CAD build for the part. Positions are in the model's coordinates, mm. A direction names the side the tool comes from. Give positions to 0.01 mm unless a question says otherwise; leave off trailing zeros. Write each loop counter-clockwise with the first axis right and the second up, starting at its lowest first coordinate (ties: lowest second). Pieces come first, ordered by that corner, then holes. Notation, with made-up numbers: (18, -36.5) - (58, -36.5) arc R19 ccw to (58, -7.5) - close; hole circle Ø1 at (17, 29). An arc over 180 degrees is marked (long way). Put each result on its own line as item: value. Start each with the question number.
1. Cut at A-A on x = 0. List the corners of the cut face in (y, z).
2. Cut at D-D on x = -32. List the corners of the cut face in (y, z).
3. Wall check: line 1 (Y direction, x = 0, z = 1.7); line 2 (X direction, y = -10, z = 3.35); line 3 (Y direction, x = 33, z = 2.85). Give the ranges that are in metal, low to high.
4. Mould opens along X. For faces 1 (the cylindrical face through (-0.56, -44.54, 2.46)), 2 (the cylindrical face through (60.14, -39.1, 2.54)), 3 (the flat face through (41, 40, 2)) say: +X half, -X half, draft (parallel to the pull), parting line (faces both ways), or undercut.
5. Drop flat-ended pins along their axis: pin 1 (18 mm diameter, centred on x = -12, y = 14, fed in from +Z); pin 2 (1.5 mm diameter, centred on x = 42.5, z = 2, fed in from +Y); pin 3 (3 mm diameter, centred on x = -9.5, z = 3.5, fed in from +Y); pin 4 (4.5 mm diameter, centred on x = 0, y = 42, fed in from +Z). Give the stop position or say it passes through.
6. Cut at C-C on y = -42. List the corners of the cut face in (x, z), and give its area (3 significant figures).
7. Cut at B-B on z = 2.25. Give the number of separate pieces and of enclosed holes in the cut face, and give its area (3 significant figures).
8. Tool access for faces 4 (the flat face through (1, 1, 0)), 5 (the flat face through (-42, 40, 2)), 6 (the flat face through (-1, 30, 3)): list every direction of +Z, -Z, +X, -X, +Y, -Y with a clear straight run to the whole face (end or side of a thin tool).
from build123d import *

# Parameters (mm, degrees)
BOSS_EXTRUDE1_DEPTH  = 5
CUT_EXTRUDE1_START   = -10
SKETCH3_R            = 2.6
CUT_EXTRUDE1_DEPTH   = 10
FILLET1_R            = 10
FILLET2_R            = 3
SKETCH4_R            = 2.6
CUT_EXTRUDE2_DEPTH   = 10
CUT_EXTRUDE3_DEPTH   = 4
CUT_EXTRUDE4_DEPTH   = 83.286086309
MIRROR2_COPY_1_DEPTH = 83.286086309


with BuildPart() as part:
    # Sketch1 → Boss-Extrude1 (new body)
    with BuildSketch(Plane.XY):
        with BuildLine():
            Line((-58, 55), (58, 55))
            ThreePointArc((58, 55), (60.121320344, 54.121320344), (61, 52))
            Line((61, 52), (61, -52))
            ThreePointArc((61, -52), (60.121320344, -54.121320344), (58, -55))
            Line((58, -55), (-58, -55))
            ThreePointArc((-58, -55), (-60.121320344, -54.121320344), (-61, -52))
            Line((-61, -52), (-61, 52))
            ThreePointArc((-61, 52), (-60.121320344, 54.121320344), (-58, 55))
        make_face()
    extrude(amount=BOSS_EXTRUDE1_DEPTH)

    # Sketch3 → Cut-Extrude1 (cut)
    with BuildSketch(Plane.XY.offset(5).offset(CUT_EXTRUDE1_START)):
        with BuildLine():
            Line((-58, 55), (-8.6, 55))
            Line((-8.6, 55), (-8.6, 59.373865289))
            Line((-8.6, 59.373865289), (-61, 59.373865289))
            Line((-61, 59.373865289), (-61, 52))
            ThreePointArc((-61, 52), (-60.121320344, 54.121320344), (-58, 55))
        make_face()
        with BuildLine():
            Line((-17.597879381, 43.752948644), (-8.6, 55))
            Line((-8.6, 55), (-58, 55))
            ThreePointArc((-58, 55), (-60.121320344, 54.121320344), (-61, 52))
            Line((-61, 52), (-61, 40))
            Line((-61, 40), (-25.40648677, 40))
            ThreePointArc((-25.40648677, 40), (-21.074657685, 40.986939655), (-17.597879381, 43.752948644))
        make_face()
        with BuildLine():
            ThreePointArc((58, 55), (60.121320344, 54.121320344), (61, 52))
            Line((61, 52), (61, 59.373865289))
            Line((61, 59.373865289), (8.6, 59.373865289))
            Line((8.6, 59.373865289), (8.6, 55))
            Line((8.6, 55), (13.480832282, 55))
            Line((13.480832282, 55), (58, 55))
        make_face()
        with BuildLine():
            ThreePointArc((17.597879381, 43.752948644), (21.074657685, 40.986939655), (25.40648677, 40))
            Line((25.40648677, 40), (61, 40))
            Line((61, 40), (61, 52))
            ThreePointArc((61, 52), (60.121320344, 54.121320344), (58, 55))
            Line((58, 55), (13.480832282, 55))
            Line((13.480832282, 55), (8.6, 55))
            Line((8.6, 55), (17.597879381, 43.752948644))
        make_face()
        with BuildLine():
            Line((61, -52), (61, -40))
            Line((61, -40), (25.40648677, -40))
            ThreePointArc((25.40648677, -40), (21.074657685, -40.986939655), (17.597879381, -43.752948644))
            Line((17.597879381, -43.752948644), (8.6, -55))
            Line((8.6, -55), (58, -55))
            ThreePointArc((58, -55), (60.121320344, -54.121320344), (61, -52))
        make_face()
        with BuildLine():
            Line((61, -59.373865289), (61, -52))
            ThreePointArc((61, -52), (60.121320344, -54.121320344), (58, -55))
            Line((58, -55), (8.6, -55))
            Line((8.6, -55), (8.6, -59.373865289))
            Line((8.6, -59.373865289), (61, -59.373865289))
        make_face()
        with BuildLine():
            Line((-58, -55), (-8.6, -55))
            Line((-8.6, -55), (-17.597879381, -43.752948644))
            ThreePointArc((-17.597879381, -43.752948644), (-21.074657685, -40.986939655), (-25.40648677, -40))
            Line((-25.40648677, -40), (-61, -40))
            Line((-61, -40), (-61, -52))
            ThreePointArc((-61, -52), (-60.121320344, -54.121320344), (-58, -55))
        make_face()
        with BuildLine():
            Line((-8.6, -59.373865289), (-8.6, -55))
            Line((-8.6, -55), (-58, -55))
            ThreePointArc((-58, -55), (-60.121320344, -54.121320344), (-61, -52))
            Line((-61, -52), (-61, -59.373865289))
            Line((-61, -59.373865289), (-8.6, -59.373865289))
        make_face()
        with Locations((0, -42)):
            Circle(SKETCH3_R)
    extrude(amount=CUT_EXTRUDE1_DEPTH, mode=Mode.SUBTRACT)

    # Fillet1
    fillet1_edges = [part.edges().sort_by_distance(p)[0] for p in [
        (-8.6, 55, 2.5),
        (8.6, 55, 2.5),
        (8.6, -55, 2.5),
        (-8.6, -55, 2.5),
    ]]
    fillet(fillet1_edges, radius=FILLET1_R)

    # Fillet2
    fillet2_edges = [part.edges().sort_by_distance(p)[0] for p in [
        (-61, -40, 2.5),
        (-61, 40, 2.5),
        (61, 40, 2.5),
        (61, -40, 2.5),
    ]]
    fillet(fillet2_edges, radius=FILLET2_R)

    # Sketch4 → Cut-Extrude2 (cut)
    with BuildSketch(Plane.XY.offset(5)):
        with Locations((0, 42)):
            Circle(SKETCH4_R)
    extrude(amount=-CUT_EXTRUDE2_DEPTH, mode=Mode.SUBTRACT)

    # Sketch5 → Cut-Extrude3 (cut)
    with BuildSketch(Plane.XY.offset(5)):
        with BuildLine():
            Line((-46, 30), (46, 30))
            ThreePointArc((46, 30), (49.535533906, 28.535533906), (51, 25))
            Line((51, 25), (51, -25))
            ThreePointArc((51, -25), (49.535533906, -28.535533906), (46, -30))
            Line((46, -30), (-46, -30))
            ThreePointArc((-46, -30), (-49.535533906, -28.535533906), (-51, -25))
            Line((-51, -25), (-51, 25))
            ThreePointArc((-51, 25), (-49.535533906, 28.535533906), (-46, 30))
        make_face()
    extrude(amount=-CUT_EXTRUDE3_DEPTH, mode=Mode.SUBTRACT)

    # Sketch6 → Cut-Extrude4 (cut, through all)
    with BuildSketch(Plane(origin=(0, 0, 0), x_dir=(-1, 0, 0), z_dir=(0, 0, -1))):
        with BuildLine():
            Line((0, 50), (-7.785066229, 50))
            ThreePointArc((-7.785066229, 50), (-12.116895314, 49.013060345), (-15.593673618, 46.247051356))
            Line((-15.593673618, 46.247051356), (-17.583467028, 43.759875465))
            ThreePointArc((-17.583467028, 43.759875465), (-21.066662425, 40.988761251), (-25.40648677, 40))
            Line((-25.40648677, 40), (-25.40648677, 70))
            Line((-25.40648677, 70), (0, 70))
            Line((0, 70), (0, 50))
        make_face()
    cut_extrude4 = extrude(amount=-CUT_EXTRUDE4_DEPTH, mode=Mode.SUBTRACT)

    # Mirror1: Cut-Extrude4 across plane
    add(cut_extrude4.mirror(Plane(origin=(0, 0, 0), x_dir=(0, 0, 1), z_dir=(1, 0, 0))), mode=Mode.SUBTRACT)

    # Mirror2: Cut-Extrude4 across plane
    add(cut_extrude4.mirror(Plane.ZX), mode=Mode.SUBTRACT)

    # Mirror2 copy 1 sketch → Mirror2 copy 1 (cut, through all)
    with BuildSketch(Plane(origin=(0, 0, 0), x_dir=(1, 0, 0), z_dir=(0, 0, -1))):
        with BuildLine():
            Line((0, 50), (-7.785066229, 50))
            ThreePointArc((-7.785066229, 50), (-12.116895314, 49.013060345), (-15.593673618, 46.247051356))
            Line((-15.593673618, 46.247051356), (-17.583467028, 43.759875465))
            ThreePointArc((-17.583467028, 43.759875465), (-21.066662425, 40.988761251), (-25.40648677, 40))
            Line((-25.40648677, 40), (-25.40648677, 70))
            Line((-25.40648677, 70), (0, 70))
            Line((0, 70), (0, 50))
        make_face()
    extrude(amount=-MIRROR2_COPY_1_DEPTH, mode=Mode.SUBTRACT)


solid = part.part
Report:
1. outline: (-50, 0) - (-44.6, 0) - (-44.6, 5) - (-50, 5) - close; (-39.4, 0) - (39.4, 0) - (39.4, 5) - (30, 5) - (30, 1) - (-30, 1) - (-30, 5) - (-39.4, 5) - close; (44.6, 0) - (50, 0) - (50, 5) - (44.6, 5) - close
2. outline: (-40, 0) - (40, 0) - (40, 5) - (30, 5) - (30, 1) - (-30, 1) - (-30, 5) - (-40, 5) - close
3. line 1: y = -50 to -44.6, -39.4 to -30, 30 to 39.4, 44.6 to 50
3. line 2: x = -61 to -51, 51 to 61
3. line 3: y = -40 to -30, 30 to 40
4. face 1: undercut
4. face 2: +X half
4. face 3: draft
5. pin 1: stops at z = 1
5. pin 2: stops at y = 40
5. pin 3: stops at y = 50
5. pin 4: passes through
6. outline: (-19.4, 0) - (-2.6, 0) - (-2.6, 5) - (-19.4, 5) - close; (2.6, 0) - (19.4, 0) - (19.4, 5) - (2.6, 5) - close
6. area: 168 mm²
7. separate pieces: 1
7. enclosed holes: 3
7. area: 4,270 mm²
8. face 4: -Z, +X, -X, +Y, -Y
8. face 5: +Z, -Z, -X, +Y
8. face 6: +Z
